Can you work these out from the model? Positions are in its coordinate system, mm. Coordinates: 2 decimals unless noted, no trailing zeros. Order: outer loops, then holes, each group sorted by start corner. A loop starts at its lowest first (then second) coordinate and runs counter-clockwise, first axis right, second up. Notation, with made-up numbers: (27.25, 22.5) - (32.25, 22.5) arc R22 ccw to (32.25, 44.5) - close; hole circle Ø10 at (-20.75, 3). An arc over 180 degrees is marked (long way). Return JSON: item names as keys, results as strings. Group by question number.
1) If I drill on line 1 along Z through (x, y) = (-32, -5); line 2 along Z through (x, y) = (-31.5, 11.5); line 3 along Y through (x, z) = (25, 56.5), over which ranges is the centre line in solid material (lowest first)?
2) For pin 1 Ø2 at (x, z) = (35, 20.5) entering from -Y; pin 2 Ø1 at (y, z) = (-25, 52.5) entering from +X; pin 3 Ø1 at (x, z) = (27, 12.5) entering from -Y, each with a flat end and sliding along its axis, tell me the tip position at first contact or that it passes through.
3) Imagine slicing it at B-B (z = 48.5). Write out the boundary of the cut face in (x, y), and give its area (3 significant figures).
4) Imagine slicing it at A-A (z = 27). Write out the boundary of the cut face in (x, y).
```python
from build123d import *

# Parameters (mm, degrees)
F1_DEPTH = 60
F2_R     = 20


with BuildPart() as f1:
    # F0 (on Top) → F1 (new body)
    with BuildSketch(Plane.XY):
        with BuildLine():
            Line((-24.4422037458, 43.6185588488), (24.4422037458, 43.6185588488))
            ThreePointArc((24.4422037458, 43.6185588488), (0, 50), (-24.4422037458, 43.6185588488))
        make_face()
        with BuildLine():
            ThreePointArc((-24.4422037458, 43.6185588488), (-25.2773595606, -43.1399477705), (50, 0))
            ThreePointArc((50, 0), (43.1399477705, 25.2773595606), (24.4422037458, 43.6185588488))
            Line((24.4422037458, 43.6185588488), (-24.4422037458, 43.6185588488))
        make_face()
    extrude(amount=F1_DEPTH)

    # F2
    f2_edges = [f1.edges().sort_by_distance(p)[0] for p in [
        (24.442204, -43.618559, 60),
    ]]
    fillet(f2_edges, radius=F2_R)


solid = f1.part
```
Calculated:
{
 "1": {"line 1": "0 to 59.86", "line 2": "0 to 59.69", "line 3": "-32.88 to 32.88"},
 "2": {"pin 1": "y = -36.66", "pin 2": "x = 38.72", "pin 3": "y = -42.4"},
 "3": {"outline": "circle Ø96.21 at (0, 0)", "area": "7,270 mm2"},
 "4": {"outline": "circle Ø100 at (0, 0)"}
}
